For this review, take the finished solid that the model builds, in its own axes (mm). Round coordinates to 2 decimals unless told otherwise and drop trailing zeros. Loops run counter-clockwise (first coordinate to the right, second up) from the corner with the lowest first, then second, coordinate; pieces in that order, holes last. Notation, with made-up numbers: M -2.5,3.25 L 7.5,3.25 A19 cw 7.5,23.25 Z; hole C 86.5,24.25 d6. An arc over 180 degrees is marked long. One line per question, with ' | ' between items. Start each with the question number.
1) We need section A-A (x = -63.5). Give the boundary of the cut face in (y, z), and give its area (3 significant figures).
2) For pin 1 Ø1.2 at (y, z) = (0, 20) entering from +X; pin 2 Ø1.5 at (x, y) = (-77, 0.5) entering from -Z; pin 3 Ø1.2 at (y, z) = (0.5, -25) entering from -X, all flat-tipped, find the tip position at first contact; note any pin that passes through.
3) For probe 1 along X at (y, z) = (-1.2, 25.5); probe 2 along Z at (x, y) = (-62, -0.25); probe 3 along X at (y, z) = (-1.3, 6), list the stretches that pass through material, from the lowest coordinate up. Write a range as from..to.
4) We need section B-B (z = 4). Give the boundary of the cut face in (x, y).
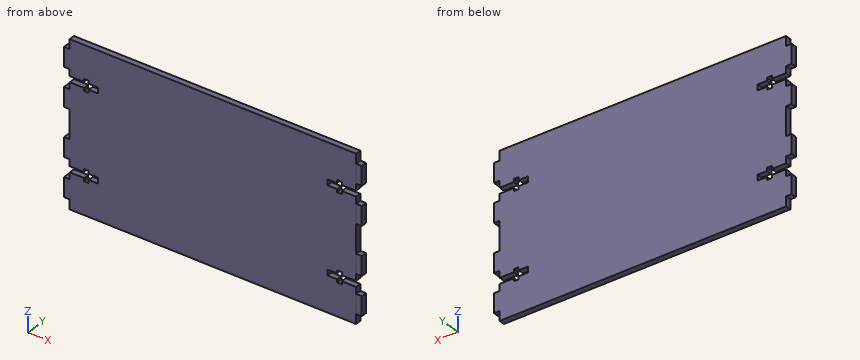
Autodesk Inventor part; units mm, degrees
ref_plane "YZ Plane" through (0, 0, 0) normal (1, 0, 0) x (0, 1, 0)
ref_plane "XZ Plane" through (0, 0, 0) normal (0, 1, 0) x (-1, 0, 0)
ref_plane "XY Plane" through (0, 0, 0) normal (0, 0, 1) x (1, 0, 0)
sketch "Эскиз1" plane through (0, 0, 0) normal (0, 1, 0) x (-1, 0, 0)
  line L0 (75.318, 42.5) -> (-75.318, 42.5)
  line L1 (-75.318, 42.5) -> (-75.318, -42.5)
  line L2 (-75.318, -42.5) -> (75.318, -42.5)
  line L3 (75.318, -42.5) -> (75.318, 42.5)
  line L4 (75.318, 42.5) -> (-75.318, -42.5) construction
  line L5 (-75.318, 42.5) -> (75.318, -42.5) construction
  point P0 (0, 0)
  dimension "d0" = 150.636
  dimension "d1" = 85
extrude "Выдавливание1" add sketch "Эскиз1" along normal mid plane 3
sketch "Эскиз3" plane through (-75.318, -1.5, 42.5) normal (-1, 0, 0) x (0, 0, 1)
  line L0 (-85, 0) -> (0, 0)
  line L1 (-80, 3) -> (-70, 3)
  line L2 (-70, 3) -> (-70, 0)
  line L3 (-70, 0) -> (-80, 0)
  line L4 (-80, 0) -> (-80, 3)
  line L5 (-80, 3) -> (-70, 0) construction
  line L6 (-70, 3) -> (-80, 0) construction
  line L7 (-60, 3) -> (-50, 3)
  line L8 (-50, 3) -> (-50, 0)
  line L9 (-50, 0) -> (-60, 0)
  line L10 (-60, 0) -> (-60, 3)
  line L11 (-60, 3) -> (-50, 0) construction
  line L12 (-50, 3) -> (-60, 0) construction
  line L13 (-35, 3) -> (-25, 3)
  line L14 (-25, 3) -> (-25, 0)
  line L15 (-25, 0) -> (-35, 0)
  line L16 (-35, 0) -> (-35, 3)
  line L17 (-35, 3) -> (-25, 0) construction
  line L18 (-25, 3) -> (-35, 0) construction
  line L19 (-15, 3) -> (-5, 3)
  line L20 (-5, 3) -> (-5, 0)
  line L21 (-5, 0) -> (-15, 0)
  line L22 (-15, 0) -> (-15, 3)
  line L23 (-15, 3) -> (-5, 0) construction
  line L24 (-5, 3) -> (-15, 0) construction
  line L25 (0, 0) -> (0, 3)
  line L26 (-85, 0) -> (-85, 3)
  point P0 (-42.5, 1.5)
  point P1 (-75, 1.5)
  point P2 (-55, 1.5)
  point P3 (-30, 1.5)
  point P4 (-10, 1.5)
  point P5 (-15, 1.5)
  point P6 (-25, 1.5)
  point P7 (-60, 1.5)
  point P8 (-35, 0)
  point P9 (-15, 0)
  dimension "d8" = 10
  dimension "d9" = 10
  dimension "d10" = 10
  dimension "d11" = 10
  dimension "d12" = 3
  dimension "d13" = 10
  dimension "d14" = 10
  dimension "d15" = 5
  dimension "d16" = 5
extrude "Выдавливание3" add sketch "Эскиз3" along normal blind 3
sketch "Эскиз4" plane through (75.318, -1.5, -42.5) normal (1, 0, 0) x (0, 0, -1)
  line L0 (-85, 3) -> (0, 3)
  line L1 (-80, 0.0026) -> (-70, 0.0026)
  line L2 (-70, 0.0026) -> (-70, 3)
  line L3 (-70, 3) -> (-80, 3)
  line L4 (-80, 3) -> (-80, 0.0026)
  line L5 (-80, 0.0026) -> (-70, 3) construction
  line L6 (-70, 0.0026) -> (-80, 3) construction
  line L7 (-60, 0.0026) -> (-50, 0.0026)
  line L8 (-50, 0.0026) -> (-50, 3)
  line L9 (-50, 3) -> (-60, 3)
  line L10 (-60, 3) -> (-60, 0.0026)
  line L11 (-60, 0.0026) -> (-50, 3) construction
  line L12 (-50, 0.0026) -> (-60, 3) construction
  line L13 (-42.5, 3) -> (-42.5, 0) construction
  line L14 (0, 0) -> (-85, 0)
  line L15 (-5, 0.0026) -> (-15, 0.0026)
  line L16 (-15, 0.0026) -> (-15, 3)
  line L17 (-15, 3) -> (-5, 3)
  line L18 (-5, 3) -> (-5, 0.0026)
  line L19 (-5, 0.0026) -> (-15, 3) construction
  line L20 (-15, 0.0026) -> (-5, 3) construction
  line L21 (-25, 0.0026) -> (-35, 0.0026)
  line L22 (-35, 0.0026) -> (-35, 3)
  line L23 (-35, 3) -> (-25, 3)
  line L24 (-25, 3) -> (-25, 0.0026)
  line L25 (-25, 0.0026) -> (-35, 3) construction
  line L26 (-35, 0.0026) -> (-25, 3) construction
  line L27 (-85, 3) -> (-85, 0)
  point P0 (-42.5, 1.5)
  point P1 (-75, 1.5013)
  point P2 (-55, 1.5013)
  point P3 (-10, 1.5013)
  point P4 (-30, 1.5013)
  point P5 (-35, 3)
  point P6 (-5, 3)
  point P7 (-15, 3)
  dimension "d19" = 10
  dimension "d24" = 20
  dimension "d29" = 5
extrude "Выдавливание4" add sketch "Эскиз4" along normal blind 3
sketch "Эскиз5" plane through (0, 1.5, 0) normal (0, 1, 0) x (1, 0, 0)
  line L0 (-75.318, 7.5) -> (-75.318, -7.5)
  line L1 (-54.4999, -2.8628) -> (-54.4999, -9.8628)
  line L2 (-54.4999, -9.8628) -> (-48.4999, -9.8628)
  line L3 (-48.4999, -9.8628) -> (-48.4999, -2.8628)
  line L4 (-48.4999, -2.8628) -> (-54.4999, -2.8628)
  line L5 (-48.4999, 3.1372) -> (-48.4999, 10.1372)
  line L6 (-48.4999, 10.1372) -> (-54.4999, 10.1372)
  line L7 (-54.4999, 10.1372) -> (-54.4999, 3.1372)
  line L8 (-54.4999, 3.1372) -> (-48.4999, 3.1372)
  line L9 (-51.4999, -2.8628) -> (-51.4999, 3.1372)
  circle A0 centre (-51.4999, 0.1372) radius 1.5
  point P0 (0, 0)
  dimension "d37" = 3
extrude "Выдавливание5" cut sketch "Эскиз5" against normal blind 3
sketch "Эскиз6" plane through (0, 1.5, 0) normal (0, 1, 0) x (1, 0, 0)
  line L0 (75.318, -27.5) -> (75.318, -17.5)
  line L1 (60.318, -24) -> (60.318, -21)
  line L2 (75.318, -21) -> (75.318, -24)
  line L3 (67.818, -25.55) -> (65.318, -25.55)
  line L4 (65.318, -19.45) -> (67.818, -19.45)
  line L5 (67.818, -19.45) -> (67.818, -21)
  line L6 (67.818, -24) -> (67.818, -25.55)
  line L7 (75.318, -24) -> (67.818, -24)
  line L8 (65.318, -24) -> (60.318, -24)
  line L9 (65.318, -25.55) -> (65.318, -24)
  line L10 (65.318, -21) -> (65.318, -19.45)
  line L11 (60.318, -21) -> (65.318, -21)
  line L12 (67.818, -21) -> (75.318, -21)
  line L13 (66.568, 0) -> (53.2147, 0) construction
  line L14 (0, -10.2584) -> (0, 8.5624) construction
  line L15 (75.318, 27.5) -> (75.318, 17.5)
  line L16 (60.318, 24) -> (60.318, 21)
  line L17 (75.318, 21) -> (75.318, 24)
  line L18 (67.818, 25.55) -> (65.318, 25.55)
  line L19 (65.318, 19.45) -> (67.818, 19.45)
  line L20 (67.818, 19.45) -> (67.818, 21)
  line L21 (67.818, 24) -> (67.818, 25.55)
  line L22 (75.318, 24) -> (67.818, 24)
  line L23 (65.318, 24) -> (60.318, 24)
  line L24 (65.318, 25.55) -> (65.318, 24)
  line L25 (65.318, 21) -> (65.318, 19.45)
  line L26 (60.318, 21) -> (65.318, 21)
  line L27 (67.818, 21) -> (75.318, 21)
  line L28 (0, 10.2584) -> (0, -8.5624) construction
  line L29 (-75.318, -27.5) -> (-75.318, -17.5)
  line L30 (-60.318, -24) -> (-60.318, -21)
  line L31 (-75.318, -21) -> (-75.318, -24)
  line L32 (-67.818, -25.55) -> (-65.318, -25.55)
  line L33 (-65.318, -19.45) -> (-67.818, -19.45)
  line L34 (-67.818, -19.45) -> (-67.818, -21)
  line L35 (-67.818, -24) -> (-67.818, -25.55)
  line L36 (-75.318, -24) -> (-67.818, -24)
  line L37 (-65.318, -24) -> (-60.318, -24)
  line L38 (-65.318, -25.55) -> (-65.318, -24)
  line L39 (-65.318, -21) -> (-65.318, -19.45)
  line L40 (-60.318, -21) -> (-65.318, -21)
  line L41 (-67.818, -21) -> (-75.318, -21)
  line L42 (-66.568, 0) -> (-53.2147, 0) construction
  line L43 (-60.318, 24) -> (-60.318, 21)
  line L44 (-65.318, 24) -> (-60.318, 24)
  line L45 (-60.318, 21) -> (-65.318, 21)
  line L46 (-65.318, 21) -> (-65.318, 19.45)
  line L47 (-65.318, 19.45) -> (-67.818, 19.45)
  line L48 (-67.818, 19.45) -> (-67.818, 21)
  line L49 (-65.318, 25.55) -> (-65.318, 24)
  line L50 (-67.818, 25.55) -> (-65.318, 25.55)
  line L51 (-67.818, 24) -> (-67.818, 25.55)
  line L52 (-67.818, 21) -> (-75.318, 21)
  line L53 (-75.318, 21) -> (-75.318, 24)
  line L54 (-75.318, 27.5) -> (-75.318, 17.5)
  line L55 (-75.318, 24) -> (-67.818, 24)
  point P0 (0, 0)
  point P1 (67.818, -23.3834)
  point P2 (67.818, 23.3834)
  point P3 (-67.818, -23.3834)
  point P4 (-67.818, 23.3834)
  point P5 (-75.318, -21)
  point P6 (75.318, -22.5)
  dimension "d38" = 6.1
  dimension "d39" = 3
  dimension "d40" = 2.5
  dimension "d41" = 15
  dimension "d42" = 1.55
  dimension "d43" = 1.55
  dimension "d44" = 1.55
  dimension "d45" = 1.55
extrude "Выдавливание6" cut sketch "Эскиз6" against normal blind 3
sketch "Эскиз7" plane through (0, 1.5, 0) normal (0, 1, 0) x (1, 0, 0)
  circle A0 centre (-51.4999, 0.1372) radius 1.5
  line L0 (-54.4999, -2.8628) -> (-48.4999, -2.8628)
  line L1 (-48.4999, -2.8628) -> (-48.4999, -9.8628)
  line L2 (-48.4999, -9.8628) -> (-54.4999, -9.8628)
  line L3 (-54.4999, -9.8628) -> (-54.4999, -2.8628)
  line L4 (-48.4999, 3.1372) -> (-54.4999, 3.1372)
  line L5 (-48.4999, 10.1372) -> (-48.4999, 3.1372)
  line L6 (-54.4999, 10.1372) -> (-48.4999, 10.1372)
  line L7 (-54.4999, 3.1372) -> (-54.4999, 10.1372)
  point P0 (0, 0)
extrude "Выдавливание8" add sketch "Эскиз7" against normal blind 3
properties part number "Нижняя часть головы_CPY"
Answers below:
1) outline: M -1.5,-42.5 L 1.5,-42.5 L 1.5,-24 L -1.5,-24 Z; M -1.5,-21 L 1.5,-21 L 1.5,21 L -1.5,21 Z; M -1.5,24 L 1.5,24 L 1.5,42.5 L -1.5,42.5 Z | area: 237 mm^2
2) pin 1: x = 75.32 | pin 2: z = -37.5 | pin 3: x = -75.32
3) probe 1: -75.32..-67.82, -65.32..65.32, 67.82..75.32 | probe 2: -42.5..-24, -21..21, 24..42.5 | probe 3: -75.32..75.32
4) outline: M -75.32,-1.5 L 75.32,-1.5 L 75.32,1.5 L -75.32,1.5 Z
